Read the model definition and answer for the solid it produces. Units are mm, in the model's axes. Face numbers are marked on the shaded views. Round coordinates to 2 decimals unless told otherwise and drop trailing zeros. Order: outer loops, then holes, each group sorted by start corner. A loop starts at its lowest first (then second) coordinate and runs counter-clockwise, first axis right, second up. Notation, with made-up numbers: (-37, 16) -> (-10, 16) arc R23 ccw to (-10, 46) -> close; hole circle Ø3 at (88.5, 27). An arc over 180 degrees is marked (long way). One line per item, written item: value. Start each with the question number.
1. Consider line 1 (Y direction, x = 44.45, z = 2.85); line 2 (X direction, y = -11.5, z = 0.85); line 3 (X direction, y = -13, z = 3.1). Determine where each line is inside the solid, lowest interval first.
2. A flat-ended cylindrical pin translates along its axis: pin 1 Ø2.5 at (x, y) = (47.625, 0) entering from +Z. Find the tip coordinate at first contact, or state that the pin passes through.
3. Section B-B (y = 0) is taken. Give the vertices of the cut face in (x, z) (3 decimals).
4. Section C-C (y = 5) is taken. Give the vertices of the cut face in (x, z).
5. Section D-D (x = 25.4) is taken. Give the vertices of the cut face in (y, z) (3 decimals).
6. The mould has two halves that part along Y. Classify the marked faces 1, 2 and 3: released by +Y, released by -Y, zero draft, split by the parting line, or undercut.
7. Section A-A (z = 2) is taken. Give the vertices of the cut face in (x, y) (3 decimals).
from build123d import *

# Parameters (mm, degrees)
SKETCH1_W              = 50.8
SKETCH1_H              = 40
BOSS_EXTRUDE1_DEPTH    = 6
SKETCH10_R             = 1.8
M3_THROUGH_DEPTH       = 55.923947418
CUT_EXTRUDE2_DEPTH     = 55.923947418
FILLET1_R              = 6.35
SKETCH8_R              = 1.5
CUT_EXTRUDE1_DEPTH     = 55.923947418
MOVE_FACE1_OUTLINE_R   = 1.8
MOVE_FACE1_OUTLINE_R_2 = 1.72
MOVE_FACE1_OUTLINE_R_3 = 1.5
MOVE_FACE1_OUTLINE_R_4 = 1.42
MOVE_FACE1_DEPTH       = 6


# Read off the part's stored shape, not the designer's step: Move Face1
with BuildPart() as part:
    # Sketch1 → Boss-Extrude1 (new body)
    with BuildSketch(Plane.XY):
        with Locations((25.4, 0)):
            Rectangle(SKETCH1_W, SKETCH1_H)
    extrude(amount=BOSS_EXTRUDE1_DEPTH)

    # Sketch10 → M3-through (cut, through all)
    with BuildSketch(Plane.XY.offset(6)):
        with Locations((44.45, 13.65)):
            Circle(SKETCH10_R)
        with Locations(Location((44.45, -13.65, 0), (0, 0, 180))):
            Circle(SKETCH10_R)
        with Locations((6.35, -13.65)):
            Circle(SKETCH10_R)
        with Locations(Location((6.35, 13.65, 0), (0, 0, 180))):
            Circle(SKETCH10_R)
    extrude(amount=-M3_THROUGH_DEPTH, mode=Mode.SUBTRACT)

    # Sketch9 → Cut-Extrude2 (cut, through all)
    with BuildSketch(Plane.XY.offset(6)):
        with BuildLine():
            Line((12.7, -8.842263568), (12.7, -20))
            Line((12.7, -20), (38.1, -20))
            Line((38.1, -20), (38.1, -8.842263568))
            ThreePointArc((38.1, -8.842263568), (25.4, 15.475), (12.7, -8.842263568))
        make_face()
    extrude(amount=-CUT_EXTRUDE2_DEPTH, mode=Mode.SUBTRACT)

    # Fillet1
    fillet1_edges = [part.edges().sort_by_distance(p)[0] for p in [
        (0, -20, 3),
        (50.8, -20, 3),
        (50.8, 20, 3),
        (0, 20, 3),
        (38.1, -20, 3),
        (38.1, -8.842263568, 3),
        (12.7, -8.842263568, 3),
        (12.7, -20, 3),
    ]]
    fillet(fillet1_edges, radius=FILLET1_R - 0.0001)  # a hair under: the kernel refuses the full size

    # Sketch8 → Cut-Extrude1 (cut, through all)
    with BuildSketch(Plane.XY.offset(6)):
        with Locations((47.625, 0)):
            Circle(SKETCH8_R)
        with Locations((3.175, 0)):
            Circle(SKETCH8_R)
    extrude(amount=-CUT_EXTRUDE1_DEPTH, mode=Mode.SUBTRACT)

    # Move Face1 outline → Move Face1 (add)
    # profile 1 of 7: a face of its own
    with BuildSketch(Plane.XY):
        with BuildLine():
            Line((-0.08, 13.65), (-0.08, -13.65))
            ThreePointArc((-0.08, -13.65), (1.803303397, -18.196696603), (6.35, -20.08))
            ThreePointArc((6.35, -20.08), (10.896696603, -18.196696603), (12.78, -13.65))
            Line((12.78, -13.65), (12.78, -10.650264081))
            ThreePointArc((12.78, -10.650264081), (12.572253945, -9.029012761), (11.962439863, -7.512523048))
            ThreePointArc((11.962439863, -7.512523048), (25.4, 15.395), (38.837560137, -7.512523048))
            ThreePointArc((38.837560137, -7.512523048), (38.227746055, -9.029012761), (38.02, -10.650264081))
            Line((38.02, -10.650264081), (38.02, -13.65))
            ThreePointArc((38.02, -13.65), (39.903303397, -18.196696603), (44.45, -20.08))
            ThreePointArc((44.45, -20.08), (48.996696603, -18.196696603), (50.88, -13.65))
            Line((50.88, -13.65), (50.88, 13.65))
            ThreePointArc((50.88, 13.65), (48.996696603, 18.196696603), (44.45, 20.08))
            Line((44.45, 20.08), (6.35, 20.08))
            ThreePointArc((6.35, 20.08), (1.803303397, 18.196696603), (-0.08, 13.65))
        make_face()
        with BuildLine():
            ThreePointArc((6.35, -20), (1.859871939, -18.140128061), (0, -13.65))
            Line((0, -13.65), (0, 13.65))
            ThreePointArc((0, 13.65), (1.859871939, 18.140128061), (6.35, 20))
            Line((6.35, 20), (44.45, 20))
            ThreePointArc((44.45, 20), (48.940128061, 18.140128061), (50.8, 13.65))
            Line((50.8, 13.65), (50.8, -13.65))
            ThreePointArc((50.8, -13.65), (48.940128061, -18.140128061), (44.45, -20))
            ThreePointArc((44.45, -20), (39.959871939, -18.140128061), (38.1, -13.65))
            Line((38.1, -13.65), (38.1, -10.650264081))
            ThreePointArc((38.1, -10.650264081), (38.305161345, -9.049183851), (38.907388316, -7.551561817))
            ThreePointArc((38.907388316, -7.551561817), (25.4, 15.475), (11.892611684, -7.551561817))
            ThreePointArc((11.892611684, -7.551561817), (12.494838655, -9.049183851), (12.7, -10.650264081))
            Line((12.7, -10.650264081), (12.7, -13.65))
            ThreePointArc((12.7, -13.65), (10.840128061, -18.140128061), (6.35, -20))
        make_face(mode=Mode.SUBTRACT)
    # profile 2 of 7: a face of its own
    with BuildSketch(Plane.XY):
        with Locations((44.45, 13.65)):
            Circle(MOVE_FACE1_OUTLINE_R)
        with Locations((44.45, 13.65)):
            Circle(MOVE_FACE1_OUTLINE_R_2, mode=Mode.SUBTRACT)
    # profile 3 of 7: a face of its own
    with BuildSketch(Plane.XY):
        with Locations((44.45, -13.65)):
            Circle(MOVE_FACE1_OUTLINE_R)
        with Locations((44.45, -13.65)):
            Circle(MOVE_FACE1_OUTLINE_R_2, mode=Mode.SUBTRACT)
    # profile 4 of 7: a face of its own
    with BuildSketch(Plane.XY):
        with Locations((6.35, -13.65)):
            Circle(MOVE_FACE1_OUTLINE_R)
        with Locations((6.35, -13.65)):
            Circle(MOVE_FACE1_OUTLINE_R_2, mode=Mode.SUBTRACT)
    # profile 5 of 7: a face of its own
    with BuildSketch(Plane.XY):
        with Locations((6.35, 13.65)):
            Circle(MOVE_FACE1_OUTLINE_R)
        with Locations((6.35, 13.65)):
            Circle(MOVE_FACE1_OUTLINE_R_2, mode=Mode.SUBTRACT)
    # profile 6 of 7: a face of its own
    with BuildSketch(Plane.XY):
        with Locations((47.625, 0)):
            Circle(MOVE_FACE1_OUTLINE_R_3)
        with Locations((47.625, 0)):
            Circle(MOVE_FACE1_OUTLINE_R_4, mode=Mode.SUBTRACT)
    # profile 7 of 7: a face of its own
    with BuildSketch(Plane.XY):
        with Locations((3.175, 0)):
            Circle(MOVE_FACE1_OUTLINE_R_3)
        with Locations((3.175, 0)):
            Circle(MOVE_FACE1_OUTLINE_R_4, mode=Mode.SUBTRACT)
    extrude(amount=MOVE_FACE1_DEPTH)


solid = part.part
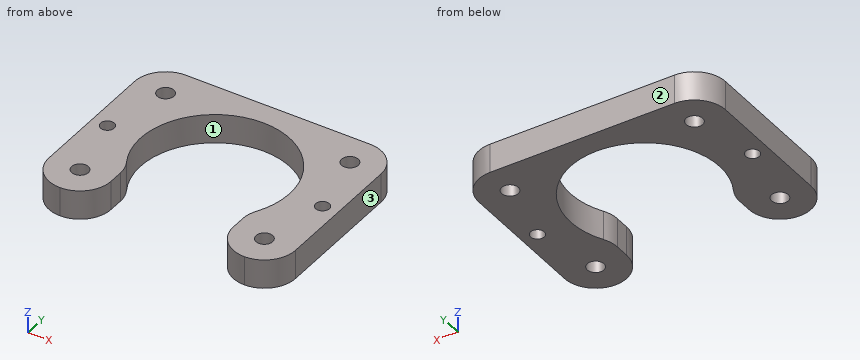
Answer:
1. line 1: -20.08 to -15.37, -11.93 to 11.93, 15.37 to 20.08
1. line 2: -0.08 to 12.78, 38.02 to 50.88
1. line 3: -0.08 to 4.76, 7.94 to 12.78, 38.02 to 42.86, 46.04 to 50.88
2. pin 1: through
3. outline: (-0.08, 0) -> (1.755, 0) -> (1.755, 6) -> (-0.08, 6) -> close; (4.595, 0) -> (10.005, 0) -> (10.005, 6) -> (4.595, 6) -> close; (40.795, 0) -> (46.205, 0) -> (46.205, 6) -> (40.795, 6) -> close; (49.045, 0) -> (50.88, 0) -> (50.88, 6) -> (49.045, 6) -> close
4. outline: (-0.08, 0) -> (10.84, 0) -> (10.84, 6) -> (-0.08, 6) -> close; (39.96, 0) -> (50.88, 0) -> (50.88, 6) -> (39.96, 6) -> close
5. outline: (15.395, 0) -> (20.08, 0) -> (20.08, 6) -> (15.395, 6) -> close
6. face 1: undercut
6. face 2: released by +Y
6. face 3: zero draft
7. outline: (-0.08, -13.65) arc R6.43 ccw to (12.78, -13.65) -> (12.78, -10.65) arc R6.43 ccw to (11.962, -7.513) arc R15.395 cw (long way) to (38.838, -7.513) arc R6.43 ccw to (38.02, -10.65) -> (38.02, -13.65) arc R6.43 ccw to (50.88, -13.65) -> (50.88, 13.65) arc R6.43 ccw to (44.45, 20.08) -> (6.35, 20.08) arc R6.43 ccw to (-0.08, 13.65) -> close; hole circle Ø2.84 at (3.175, 0); hole circle Ø3.44 at (6.35, -13.65); hole circle Ø3.44 at (6.35, 13.65); hole circle Ø3.44 at (44.45, -13.65); hole circle Ø3.44 at (44.45, 13.65); hole circle Ø2.84 at (47.625, 0)
